Here's how the part is built. I have some questions about the finished solid (model axes, mm). A direction names the side the tool comes from. Round coordinates to 2 decimals unless told otherwise and drop trailing zeros. Order: outer loops, then holes, each group sorted by start corner. A loop starts at its lowest first (then second) coordinate and runs counter-clockwise, first axis right, second up.
```python
from build123d import *

# Parameters (mm, degrees)
SKETCH2_R                = 30
BOSS_EXTRUDE1_DEPTH      = 1
BOSS_EXTRUDE2_DEPTH      = 1
BOSS_EXTRUDE2_DEPTH_BACK = 2
SCALE1_SCALE             = 2
BOSS_EXTRUDE3_DEPTH      = 5
BOSS_EXTRUDE3_DEPTH_BACK = 11
SKETCH5_W                = 20
SKETCH5_H                = 10
FILLET1_R                = 10
FILLET2_R                = 10
FILLET3_R                = 10
CUT_EXTRUDE3_DEPTH       = 3
SKETCH13_R               = 1.25
BOSS_EXTRUDE4_DEPTH      = 2
SCALE2_SCALE             = 0.8


with BuildPart() as part:
    # Sketch2 → Boss-Extrude1 (new body)
    with BuildSketch(Plane(origin=(0, 0, 0), x_dir=(1, 0, 0), z_dir=(0, 1, 0))):
        with Locations(Location((0, 0, 0), (0, 0, 270))):
            Circle(SKETCH2_R)
    extrude(amount=BOSS_EXTRUDE1_DEPTH)

    # Sketch3 → Boss-Extrude2 (add, two sides: drawn at the far end of the back side and taken through both)
    with BuildSketch(Plane(origin=(0, 1, 0), x_dir=(1, 0, 0), z_dir=(0, 1, 0)).offset(-BOSS_EXTRUDE2_DEPTH_BACK)):
        with BuildLine():
            Line((-14.290451106, -26.37769905), (-14.290451106, -34.782711282))
            Line((-14.290451106, -34.782711282), (-2.11058873, -34.782711282))
            ThreePointArc((-2.11058873, -34.782711282), (27.5349766, -21.80785282), (38.117480018, 8.773466924))
            ThreePointArc((38.117480018, 8.773466924), (39.698443789, 14.79025178), (44.684067377, 18.511098982))
            Line((44.684067377, 18.511098982), (87.64168842, 18.511098982))
            ThreePointArc((87.64168842, 18.511098982), (86.998038921, 24.281089627), (85.098734122, 29.767410617))
            Line((85.098734122, 29.767410617), (39.674176802, 29.767410617))
            Line((39.674176802, 29.767410617), (25.714146622, 33.856712387))
            ThreePointArc((25.714146622, 33.856712387), (1.610609717, 36.463459714), (-21.899290339, 30.542292401))
            ThreePointArc((-21.899290339, 30.542292401), (-21.763636639, 25.798277328), (-21.355544159, 21.069901131))
            Line((-21.355544159, 21.069901131), (6.360164673, 21.069901131))
            Line((6.360164673, 21.069901131), (6.867267346, 20.563219729))
            ThreePointArc((6.867267346, 20.563219729), (12.505714755, -10.216879454), (-14.290451106, -26.37769905))
        make_face()
    extrude(amount=BOSS_EXTRUDE2_DEPTH + BOSS_EXTRUDE2_DEPTH_BACK)


with BuildPart() as part_1:
    # Scale1: scaled about (18.795730072, 0.5, -7.565232671)
    add(part.part.scale(SCALE1_SCALE).moved(Location((-18.795730072, -0.5, 7.565232671))))

    # Sketch5 → Boss-Extrude3 (add, two sides: drawn at the far end of the back side and taken through both)
    with BuildSketch(Plane.XY.offset(-29.456965293).offset(-BOSS_EXTRUDE3_DEPTH_BACK)):
        with Locations((127.136416626, 0.749159319)):
            Rectangle(SKETCH5_W, SKETCH5_H)
    extrude(amount=BOSS_EXTRUDE3_DEPTH + BOSS_EXTRUDE3_DEPTH_BACK)

    # Fillet1
    fillet1_edges = [part_1.edges().sort_by_distance(p)[0] for p in [
        (-47.376632285, 0.5, 77.130655235),
    ]]
    fillet(fillet1_edges, radius=FILLET1_R)

    # Fillet2
    fillet2_edges = [part_1.edges().sort_by_distance(p)[0] for p in [
        (-62.59431075, 0.5, -53.519352131),
    ]]
    fillet(fillet2_edges, radius=FILLET2_R)

    # Fillet3
    fillet3_edges = [part_1.edges().sort_by_distance(p)[0] for p in [
        (156.487646768, 0.5, -29.456965293),
    ]]
    fillet(fillet3_edges, radius=FILLET3_R)

    # Sketch12 → Cut-Extrude3 (cut)
    with BuildSketch(Plane.XY.offset(-24.456965293)):
        Polygon((124.436416626, 0.749159319), (124.145484747, 0.961193849), (124.186719528, 1.287600755), (124.521242091, 1.420622015), (124.292181215, 1.698346906), (124.413294627, 2.004244466), (124.770388589, 2.049894239), (124.617591455, 2.375859016), (124.810973495, 2.64202656), (125.168201332, 2.597436505), (125.101268743, 2.951159601), (125.354768508, 3.160872845), (125.689684279, 3.028844718), (125.712821858, 3.38810041), (126.010511024, 3.528182299), (126.302070741, 3.317011913), (126.413824668, 3.659226845), (126.736998331, 3.720875519), (126.966882223, 3.443831486), (127.160230587, 3.747503035), (127.488582557, 3.72684488), (127.642346175, 3.401334896), (127.905140188, 3.647382262), (128.218038903, 3.545715307), (128.286020713, 3.192192361), (128.601748061, 3.365155483), (128.879532943, 3.188867836), (128.857461398, 2.829545075), (129.20628377, 2.918556044), (129.431500575, 2.678724506), (129.32076251, 2.3361795), (129.680762114, 2.33564543), (129.839259641, 2.047339499), (129.646813137, 1.743095611), (129.995369874, 1.653050059), (130.07718914, 1.334385057), (129.815126319, 1.08755905), (130.130339086, 0.913659908), (130.130339086, 0.58465873), (129.815126319, 0.410759589), (130.07718914, 0.163933581), (129.995369874, -0.15473142), (129.646813137, -0.244776973), (129.839259641, -0.549020861), (129.680762114, -0.837326791), (129.32076251, -0.837860862), (129.431500575, -1.180405868), (129.20628377, -1.420237405), (128.857461398, -1.331226436), (128.879532943, -1.690549198), (128.601748061, -1.866836845), (128.286020713, -1.693873722), (128.218038903, -2.047396669), (127.905140188, -2.149063624), (127.642346175, -1.903016258), (127.488582557, -2.228526242), (127.136416626, -2.250840681), (126.966882223, -1.945512848), (126.736998331, -2.22255688), (126.379896011, -2.153886764), (126.302070741, -1.818693275), (126.010511024, -2.029863661), (125.712821858, -1.889781772), (125.689684279, -1.53052608), (125.354768508, -1.662554207), (125.101268743, -1.452840963), (125.168201332, -1.099117867), (124.810973495, -1.143707922), (124.617591455, -0.877540378), (124.770388589, -0.551575601), (124.413294627, -0.505925827), (124.292181215, -0.200028268), (124.521242091, 0.077696624), (124.186719528, 0.210717883), (124.145484747, 0.537124789), align=None)
    extrude(amount=-CUT_EXTRUDE3_DEPTH, mode=Mode.SUBTRACT)

    # Sketch13 → Boss-Extrude4 (add)
    with BuildSketch(Plane.XY.offset(-27.456965293)):
        with Locations((127.136416626, 0.749159319)):
            Circle(SKETCH13_R)
    extrude(amount=BOSS_EXTRUDE4_DEPTH)


with BuildPart() as part_2:
    # Scale2: scaled about (21.037420475, 0.509511918, -8.126150546)
    add(part_1.part.scale(SCALE2_SCALE).moved(Location((4.207484095, 0.101902384, -1.625230109))))


solid = part_2.part
```
1. If we section it at A-A, the plane x = 111: Write out the boundary of the cut face in (y, z).
Evaluation:
outline: (-3.3, -33.99) - (-1.9, -33.99) - (-1.9, -43.2) - (2.9, -43.2) - (2.9, -33.99) - (4.7, -33.99) - (4.7, -21.19) - (-3.3, -21.19) - close
2. On a 3-axis mill with a long thin cutter (end or side, diameter ignored), from which of +Z, -Z, +X, -X, +Y, -Y can I reach the whole of each face in a straight line? I mean faces 4 (the flat face through (89, 0, -43.201)), 5 (the flat face through (-22, 1.302, 8)), 6 (the cylindrical face through (-45.466, 0.468, -34.122)). Say none if no direction works.
Evaluation:
face 4: -Z, +X, +Y, -Y
face 5: -X, +Y
face 6: -X, +Y, -Y
3. If we mould it in two halves opening along Z, with no side actions, what happens to faces 1 (the cylindrical face through (126.791, 0.536, -28.326)), 2 (the flat face through (104, 3, -21.191)), 3 (the cylindrical face through (9.48, 2.09, 20.09))? For each: released by +Z, released by -Z, zero draft, split by the parting line, or undercut.
Evaluation:
face 1: split by the parting line
face 2: released by +Z
face 3: undercut
4. If we section it at C-C, the plane x = -3: Write out the boundary of the cut face in (y, z), and give its area (3 significant figures).
Evaluation:
outline: (-1.9, -54.15) - (2.9, -54.15) - (2.9, -29.28) - (1.3, -29.28) - (1.3, 36.69) - (2.9, 36.69) - (2.9, 59.1) - (-1.9, 59.1) - (-1.9, 36.69) - (-0.3, 36.69) - (-0.3, -29.28) - (-1.9, -29.28) - close
area: 332 mm2
5. If we section it at D-D, the plane x = 88: Write out the boundary of the cut face in (y, z), and give its area (3 significant figures).
Evaluation:
outline: (-1.9, -43.2) - (2.9, -43.2) - (2.9, -25.19) - (-1.9, -25.19) - close
area: 86.4 mm2
6. I need wall thicknesses on probe 1 along Y at (x, z) = (66, -42.5); probe 2 along Y at (x, z) = (1, -17); probe 3 along Z at (x, y) = (104, 4.25). Which ranges of each line are inside material? Lowest first, please.
Evaluation:
probe 1: y = -1.9 to 2.9
probe 2: y = -0.3 to 1.3
probe 3: z = -33.99 to -21.19
7. I'm going to push flat-ended pins straight in: P1, Ø2.5, axis at x = 118.5, y = 0, coming from the +Z side; P2, Ø3, axis at x = 19.5, y = 2, coming from the -Z side; P3, Ø0.9, axis at x = 103.5, y = 4, coming from the -Z side. Where does each tip first touch, or does it pass through?
Evaluation:
P1: stops at z = -25.19
P2: stops at z = -52.59
P3: stops at z = -33.99
8. If we section it at B-B, the plane z = 34: Write out the boundary of the cut face in (x, y).
Evaluation:
outline: (-48.64, -0.3) - (-0.01, -0.3) - (-0.01, -1.9) - (37.64, -1.9) - (37.64, 2.9) - (-0.01, 2.9) - (-0.01, 1.3) - (-48.64, 1.3) - close
